Input: part model. Units: mm. Frame: model coordinates. Face numbers are marked on the shaded views. A direction names the side the tool comes from. Coordinates: 2 decimals unless noted, no trailing zeros. Loops run counter-clockwise (first coordinate to the right, second up) from the corner with the lowest first, then second, coordinate; pieces in that order, holes last. Notation, with made-up numbers: (64, 35.5) -> (117, 35.5) arc R10 ccw to (117, 49.5) -> close; hole circle Ø11 at (11.5, 13). An arc over 180 degrees is marked (long way). Answer as a JSON object with one key per item and string values.
from build123d import *

# Parameters (mm, degrees)
ESQUISSE2_R                  = 12.5
ENL_V_MAT_EXTRU_1_DEPTH      = 47
R_P_TITION_CIRCULAIRE1_COUNT = 3
R_P_TITION_CIRCULAIRE2_COUNT = 3


with BuildPart() as part:
    # Esquisse1 → Révolution1 (revolve)
    with BuildSketch(Plane.XY, mode=Mode.PRIVATE) as r_volution1_sk:
        Polygon((0, 0), (23, 0), (23, 46), (15, 46), (15, 33), (16.37708167, 30.614824582), (16.37708167, 18.385175418), (15, 16), (15, 6), (0, 6), align=None)
    revolve(r_volution1_sk.sketch.rotate(Axis((0, 6, 0), (0, -1, 0)), 90), axis=Axis((0, 6, 0), (0, -1, 0)))  # turned: the seam where the file's is

    # Esquisse2 → Enlèv. mat.-Extru.1 (cut, through all)
    with BuildSketch(Plane.XZ):
        with Locations(Location((0, 0, 0), (0, 0, 270))):  # turned: the seam where the file's is
            Circle(ESQUISSE2_R)
    extrude(amount=-ENL_V_MAT_EXTRU_1_DEPTH, mode=Mode.SUBTRACT)

    # Esquisse3 → Trou taraudé M51 (revolve, cut)
    with BuildSketch(Plane(origin=(0, 0, 19), x_dir=(0, 0, -1), z_dir=(1, 0, 0))):
        Polygon((0, 0), (0, 13.2618073), (2.1, 12), (2.1, 0), align=None)
    trou_taraud_m51 = revolve(axis=Axis((0, -6.35, 19), (0, 1, 0)), mode=Mode.SUBTRACT)

    # Répétition circulaire1: Trou taraudé M51 ×3 about axis
    r_p_tition_circulaire1_axis = Axis((0, 0, 0), (0, 1, 0))
    for i in range(1, R_P_TITION_CIRCULAIRE1_COUNT):
        add(trou_taraud_m51.rotate(r_p_tition_circulaire1_axis, i * 360 / R_P_TITION_CIRCULAIRE1_COUNT), mode=Mode.SUBTRACT)

    # Esquisse7 → Trou taraudé M31 (revolve, cut)
    with BuildSketch(Plane(origin=(0, 46, 19), x_dir=(0, 0, 1), z_dir=(1, 0, 0))):
        Polygon((0, 0), (0, 9.251075774), (1.25, 8.5), (1.25, 0), align=None)
    trou_taraud_m31 = revolve(axis=Axis((0, 52.35, 19), (0, -1, 0)), mode=Mode.SUBTRACT)

    # Répétition circulaire2: Trou taraudé M31 ×3 about axis
    r_p_tition_circulaire2_axis = Axis((0, 0, 0), (0, 1, 0))
    for i in range(1, R_P_TITION_CIRCULAIRE2_COUNT):
        add(trou_taraud_m31.rotate(r_p_tition_circulaire2_axis, i * 360 / R_P_TITION_CIRCULAIRE2_COUNT), mode=Mode.SUBTRACT)


solid = part.part
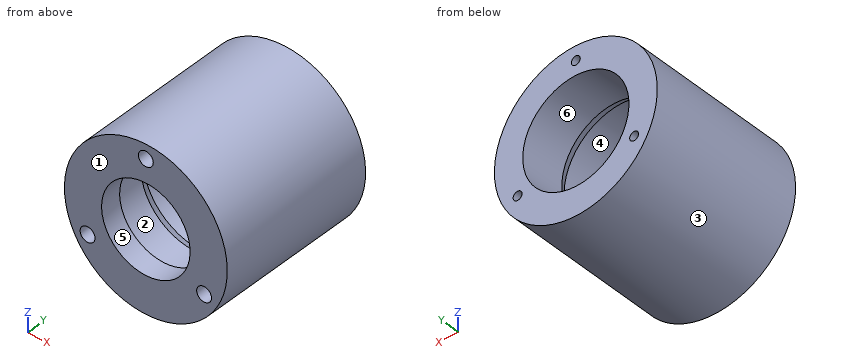
1. Section query C-C (y = 27). Return loops of the section in (x, z), plus the area to 3 significant figures.
Reply:
{"outline": "circle Ø46 at (0, 0); hole circle Ø32.75 at (0, 0)", "area": "819 mm2"}
2. Mould query, pull axis X, two halves, no side actions, for the marked faces 1, 2 and 3. Classes: pulls with the +X half, pulls with the -X half, needs draft (parallel to the pull), parting line crosses it, or undercut.
Reply:
{"face 1": "needs draft", "face 2": "undercut", "face 3": "parting line crosses it"}
3. Section query D-D (x = -19.5). Return loops of the section in (y, z).
Reply:
{"outline": "(0, -12.2) -> (46, -12.2) -> (46, 12.2) -> (0, 12.2) -> close"}
4. Section query B-B (y = 40). Return loops of the section in (x, z) (3 decimals), plus the area to 3 significant figures.
Reply:
{"outline": "circle Ø46 at (0, 0); hole circle Ø2.5 at (-16.454, -9.5); hole circle Ø30 at (0, 0); hole circle Ø2.5 at (0, 19); hole circle Ø2.5 at (16.454, -9.5)", "area": "940 mm2"}
5. Line query: line 1 along X through (y, z) = (9.25, -9.5); line 2 along X through (y, z) = (4.5, -11); line 3 along Y through (x, z) = (4.5, 13). Output: solid intervals per line, ascending.
Reply:
{"line 1": "x = -20.95 to -18.55, -14.35 to -11.61, 11.61 to 14.35, 18.55 to 20.95", "line 2": "x = -20.2 to -17.92, -14.98 to -5.94, 5.94 to 14.98, 17.92 to 20.2", "line 3": "y = 0 to 6"}
6. Access query for the marked faces 4, 5 and 6. Directions: +Z, -Z, +X, -X, +Y, -Y. A direction counts if a zero-diameter tool reaches every point of the face in a straight line with its end or side. Return the directions, or none.
Reply:
{"face 4": "none", "face 5": "+Y, -Y", "face 6": "+Y"}
7. Section query A-A (z = 0). Return loops of the section in (x, y).
Reply:
{"outline": "(-23, 0) -> (-12.5, 0) -> (-12.5, 6) -> (-15, 6) -> (-15, 16) -> (-16.38, 18.39) -> (-16.38, 30.61) -> (-15, 33) -> (-15, 46) -> (-23, 46) -> close; (12.5, 0) -> (23, 0) -> (23, 46) -> (15, 46) -> (15, 33) -> (16.38, 30.61) -> (16.38, 18.39) -> (15, 16) -> (15, 6) -> (12.5, 6) -> close"}
8. Pin query (flat end, axial travel): P1, Ø2, axis at x = 16.5, y = 29.5, coming from the -Z side; P2, Ø18, axis at x = 0, z = 0, coming from the +Y side; P3, Ø1, axis at x = -15, y = 33, coming from the -Z side; P4, Ø6, axis at x = 8, y = 23.5, coming from the -Z side. Return the tip coordinate at first contact, or that it passes through.
Reply:
{"P1": "stops at z = -16.99", "P2": "passes through", "P3": "stops at z = -17.85", "P4": "stops at z = -22.45"}
